Input: part model. Units: mm. Frame: model coordinates. Face numbers are marked on the shaded views. A direction names the side the tool comes from. Coordinates: 2 decimals unless noted, no trailing zeros. Loops run counter-clockwise (first coordinate to the right, second up) from the corner with the lowest first, then second, coordinate; pieces in that order, holes last. Notation, with made-up numbers: (57, 11.25) -> (106, 11.25) arc R23 cw to (106, 29.25) -> close; hole circle Ø5 at (16, 76.25). An arc over 180 degrees is marked (long way). Answer as a JSON object with one key per item and string values.
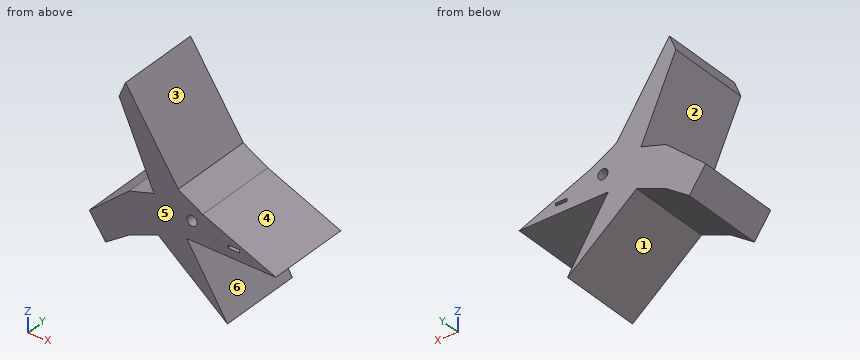
from build123d import *

# Parameters (mm, degrees)
F1_DEPTH = 50.8
F2_R     = 3.061236
F3_DEPTH = 50.8
F4_W     = 6.747894
F4_H     = 1.79878
F5_DEPTH = 50.8


with BuildPart() as f1:
    # F0 (on Front) → F1 (new body)
    with BuildSketch(Plane.XZ):
        Polygon((8.592959, 2.100501), (62.442172, 1.718592), (18.331647, 19.859284), (3.437185, 28.261289), (-28.452244, 76.572813), (-32.311786, 67.188031), (-11.266325, 19.859284), (-26.351742, 15.085418), (-50.412029, -5.72864), (-40.482387, -20.050241), (-26.351742, -10.252995), (-8.592959, -3.055275), (33.22611, -37.045203), align=None)
    extrude(amount=F1_DEPTH)

    # F2 (on face) → F3 (cut)
    with BuildSketch(Plane.XZ.offset(50.8)):
        with Locations((11.83919, 13.557781)):
            Circle(F2_R)
    extrude(amount=-F3_DEPTH, mode=Mode.SUBTRACT)

    # F4 (on face) → F5 (cut)
    with BuildSketch(Plane.XZ.offset(50.8)):
        with Locations((36.995076, 7.709399)):
            Rectangle(F4_W, F4_H)
    extrude(amount=-F5_DEPTH, mode=Mode.SUBTRACT)


solid = f1.part
1. Section query C-C (y = -21). Return loops of the section in (x, z).
Reply:
{"outline": "(-50.41, -5.73) -> (-40.48, -20.05) -> (-26.35, -10.25) -> (-8.59, -3.06) -> (33.23, -37.05) -> (8.59, 2.1) -> (62.44, 1.72) -> (18.33, 19.86) -> (3.44, 28.26) -> (-28.45, 76.57) -> (-32.31, 67.19) -> (-11.27, 19.86) -> (-26.35, 15.09) -> close; hole circle Ø6.12 at (11.84, 13.56); hole (33.62, 6.81) -> (40.37, 6.81) -> (40.37, 8.61) -> (33.62, 8.61) -> close"}
2. Pin query (flat end, axial travel): P1, Ø2, axis at y = -26, z = 6.5, coming from the -X side; P2, Ø1.5, axis at y = -19.5, z = 8, coming from the -X side; P3, Ø2, axis at y = -24, z = 8, coming from the +X side; P4, Ø3.5, axis at x = 11.84, z = 13.56, coming from the -Y side. Return the tip coordinate at first contact, or that it passes through.
Reply:
{"P1": "stops at x = -37.43", "P2": "stops at x = -35.41", "P3": "stops at x = 49.6", "P4": "passes through"}
3. Section query D-D (x = 11.5). Return loops of the section in (y, z).
Reply:
{"outline": "(-50.8, -19.39) -> (0, -19.39) -> (0, -2.52) -> (-50.8, -2.52) -> close; (-50.8, 2.08) -> (0, 2.08) -> (0, 10.52) -> (-50.8, 10.52) -> close; (-50.8, 16.6) -> (0, 16.6) -> (0, 23.71) -> (-50.8, 23.71) -> close"}
4. Access query for the marked faces 1, 2 and 3. Directions: +Z, -Z, +X, -X, +Y, -Y. A direction counts if a zero-diameter tool reaches every point of the face in a straight line with its end or side. Return the directions, or none.
Reply:
{"face 1": "-Z, +Y, -Y", "face 2": "-X, +Y, -Y", "face 3": "+Z, +X, +Y, -Y"}
5. Section query B-B (z = -7.5). Return loops of the section in (x, y).
Reply:
{"outline": "(-49.18, -50.8) -> (-19.56, -50.8) -> (-19.56, 0) -> (-49.18, 0) -> close; (-3.12, -50.8) -> (14.63, -50.8) -> (14.63, 0) -> (-3.12, 0) -> close"}
6. Mould query, pull axis Z, two halves, no side actions, for the marked faces 4, 5 and 6. Classes: pulls with the +Z half, pulls with the -Z half, needs draft (parallel to the pull), parting line crosses it, or undercut.
Reply:
{"face 4": "pulls with the +Z half", "face 5": "needs draft", "face 6": "undercut"}
7. Section query A-A (x = 27.5). Return loops of the section in (y, z).
Reply:
{"outline": "(-50.8, -32.39) -> (0, -32.39) -> (0, -27.95) -> (-50.8, -27.95) -> close; (-50.8, 1.97) -> (0, 1.97) -> (0, 16.09) -> (-50.8, 16.09) -> close"}
8. Line query: line 1 along Z through (x, y) = (-20, -31); line 2 along Z through (x, y) = (36, -26); line 3 along X through (y, z) = (-42, -4.5). Output: solid intervals per line, ascending.
Reply:
{"line 1": "z = -7.68 to 17.1, 39.5 to 63.77", "line 2": "z = 1.91 to 6.81, 8.61 to 12.59", "line 3": "x = -48.99 to -12.16, -6.82 to 12.75"}
